```python
from build123d import *

# Parameters (mm, degrees)
SKETCH1_W                       = 60
SKETCH1_H                       = 15
BOSS_EXTRUDE1_DEPTH             = 5
BOSS_EXTRUDE2_REACH             = 33.325
SKETCH2_R                       = 12.5
BOSS_EXTRUDE2_DIRECTION_2_REACH = 33.325
SKETCH3_W                       = 55
SKETCH3_H                       = 2
CUT_EXTRUDE1_DEPTH              = 56.082201073
DRAFT1_START                    = 7.751401292
DRAFT1_DEPTH                    = 3.248598708


with BuildPart() as part:
    # Sketch1 → Boss-Extrude1 (new body)
    with BuildSketch(Plane(origin=(0, 0, 0), x_dir=(1, 0, 0), z_dir=(0, 1, 0))):
        Rectangle(SKETCH1_W, SKETCH1_H)
    extrude(amount=BOSS_EXTRUDE1_DEPTH)

    # Boss-Extrude2: up to this face of the body (flat: up to its plane)
    boss_extrude2_end = Plane(part.part.faces().sort_by_distance((0, 2.5, 7.5))[0])
    # Sketch2 → Boss-Extrude2 (add, up to the picked face)
    with BuildSketch(Plane.XY, mode=Mode.PRIVATE) as boss_extrude2_sk1:
        with BuildLine():
            Line((-17.13013706, 5), (-14.942920471, 30))
            ThreePointArc((-14.942920471, 30), (0, 43.692663859), (14.942920471, 30))
            Line((14.942920471, 30), (17.13013706, 5))
            Line((17.13013706, 5), (-17.13013706, 5))
        make_face()
        with Locations(Location((0, 28.692663859, 0), (0, 0, 180))):
            Circle(SKETCH2_R, mode=Mode.SUBTRACT)
    boss_extrude2_tool1 = split(extrude(boss_extrude2_sk1.sketch, amount=BOSS_EXTRUDE2_REACH, mode=Mode.PRIVATE), bisect_by=boss_extrude2_end, keep=Keep.BOTH, mode=Mode.PRIVATE)
    add(boss_extrude2_tool1.solids().sort_by(Axis((15.521689, 17.454957, 0), (0, 0, 1)))[0])

    # Boss-Extrude2 direction 2: up to this face of the body (flat: up to its plane)
    boss_extrude2_direction_2_end = Plane(part.part.faces().sort_by_distance((0, 2.5, -7.5))[0])
    # Sketch2 → Boss-Extrude2 direction 2 (add, up to the picked face)
    with BuildSketch(Plane.XY, mode=Mode.PRIVATE) as boss_extrude2_direction_2_sk1:
        with BuildLine():
            Line((-17.13013706, 5), (-14.942920471, 30))
            ThreePointArc((-14.942920471, 30), (0, 43.692663859), (14.942920471, 30))
            Line((14.942920471, 30), (17.13013706, 5))
            Line((17.13013706, 5), (-17.13013706, 5))
        make_face()
        with Locations(Location((0, 28.692663859, 0), (0, 0, 180))):
            Circle(SKETCH2_R, mode=Mode.SUBTRACT)
    boss_extrude2_direction_2_tool1 = split(extrude(boss_extrude2_direction_2_sk1.sketch, amount=-BOSS_EXTRUDE2_DIRECTION_2_REACH, mode=Mode.PRIVATE), bisect_by=boss_extrude2_direction_2_end, keep=Keep.BOTH, mode=Mode.PRIVATE)
    add(boss_extrude2_direction_2_tool1.solids().sort_by(Axis((15.521689, 17.454957, 0), (0, 0, -1)))[0])

    # Sketch3 → Cut-Extrude1 (cut, through all)
    with BuildSketch(Plane.XY.offset(7.5)):
        Rectangle(SKETCH3_W, SKETCH3_H)
    extrude(amount=-CUT_EXTRUDE1_DEPTH, mode=Mode.SUBTRACT)

    # Draft1: read off the stored shape, not the designer's step
    # Draft1 outline → Draft1 (cut)
    with BuildSketch(Plane(origin=(0, 0, 0), x_dir=(1, 0, 0), z_dir=(0, 0.05233595624294388, 0.9986295347545738)).offset(DRAFT1_START)):
        with BuildLine():
            add(Edge.make_bspline(
                [(14.942920471, 29.634936652), (13.74496761, 43.346391583), (0, 43.346391583), (-13.74496761, 43.346391583), (-14.942920471, 29.634936652)],
                knots=[4.799655443, 4.799655443, 4.799655443, 6.283185307, 6.283185307, 7.766715171, 7.766715171, 7.766715171], degree=2, weights=[1, 0.737277337, 1, 0.737277337, 1]))
            Line((-14.942920471, 29.634936652), (-17.13013706, 4.600628002))
            Line((-17.13013706, 4.600628002), (17.13013706, 4.600628002))
            Line((17.13013706, 4.600628002), (14.942920471, 29.634936652))
        make_face()
    extrude(amount=DRAFT1_DEPTH, mode=Mode.SUBTRACT)


solid = part.part
```
Can you work these out from the model? Positions are in its coordinate system, mm. A direction names the side the tool comes from. Coordinates: 2 decimals unless noted, no trailing zeros. Order: outer loops, then holes, each group sorted by start corner. A loop starts at its lowest first (then second) coordinate and runs counter-clockwise, first axis right, second up. Notation, with made-up numbers: (19.5, -6) - (75.5, -6) arc R21 ccw to (75.5, 4) - close; hole circle Ø7 at (18.5, 48.25). An arc over 180 degrees is marked (long way). Answer in a Markdown table with one row per item.
1. Suppose I cut it at C-C (z = 3.25). Please give me the cut outline in (x, y).
Reply:
| item | result |
|---|---|
| outline | (-30, 0) - (-27.5, 0) - (-27.5, 1) - (27.5, 1) - (27.5, 0) - (30, 0) - (30, 5) - (17.13, 5) - (14.94, 30) arc R15 ccw to (-14.94, 30) - (-17.13, 5) - (-30, 5) - close; hole circle Ø25 at (0, 28.69) |
2. Suppose I cut it at B-B (y = 35.5). Please give me the cut outline in (x, z), and give its area (3 significant figures).
Reply:
| item | result |
|---|---|
| outline | (-13.37, -7.5) - (-10.48, -7.5) - (-10.48, 5.9) - (-13.37, 5.9) - close; (10.48, -7.5) - (13.37, -7.5) - (13.37, 5.9) - (10.48, 5.9) - close |
| area | 77.3 mm^2 |
3. For pin 1 (1 mm diameter, centred on y = 26, z = -4, fed in from -X); pin 2 (1.5 mm diameter, centred on x = -22.5, z = 2, fed in from -Y); pin 3 (8 mm diameter, centred on x = 10.5, z = 4, fed in from +Y), each with a flat end and sliding along its axis, tell me the tip position at first contact or that it passes through.
Reply:
| item | result |
|---|---|
| pin 1 | stops at x = -15.34 |
| pin 2 | stops at y = 1 |
| pin 3 | stops at y = 42.21 |
4. Suppose I cut it at D-D (x = 0). Please give me the cut outline in (y, z).
Reply:
| item | result |
|---|---|
| outline | (1, -7.5) - (16.19, -7.5) - (16.19, 6.91) - (5, 7.5) - (1, 7.5) - close; (41.19, -7.5) - (43.69, -7.5) - (43.69, 5.47) - (41.19, 5.6) - close |
5. If I drill on line 1 along Y through (x, z) = (0, 2.25); line 2 along X through (y, z) = (29, 4.75); line 3 along Y through (x, z) = (-2, -6.25), over which ranges is the centre line in solid material (lowest first)?
Reply:
| item | result |
|---|---|
| line 1 | y = 1 to 16.19, 41.19 to 43.69 |
| line 2 | x = -15.03 to -12.5, 12.5 to 15.03 |
| line 3 | y = 1 to 16.35, 41.03 to 43.56 |
6. Suppose I cut it at A-A (x = 11). Please give me the cut outline in (y, z).
Reply:
| item | result |
|---|---|
| outline | (1, -7.5) - (22.76, -7.5) - (22.76, 6.57) - (5, 7.5) - (1, 7.5) - close; (34.63, -7.5) - (38.89, -7.5) - (38.89, 5.72) - (34.63, 5.95) - close |
7. For faces 4 (the flat face through (23, 5, 0)), 5 (the flat face through (-24, 5, 0)), 6 (the flat face through (-29, 0, 0)), which set-ups out of +Z, -Z, +X, -X, +Y, -Y let a thin tool reach every point of the face, with its end or its side?
Reply:
| item | result |
|---|---|
| face 4 | +Z, -Z, +X, +Y |
| face 5 | +Z, -Z, -X, +Y |
| face 6 | +Z, -Z, +X, -X, -Y |
8. If we mould it in two halves opening along X, with no side actions, what happens to faces 1 (the flat face through (0, 3, 7.5)), 2 (the cylindrical face through (-0.31, 43.69, -0.56)), 3 (the flat face through (0, 1, 0))? For each: pulls with the +X half, pulls with the -X half, needs draft (parallel to the pull), parting line crosses it, or undercut.
Reply:
| item | result |
|---|---|
| face 1 | needs draft |
| face 2 | parting line crosses it |
| face 3 | undercut |
